Can you work these out from the model? Positions are in its coordinate system, mm. Face numbers are marked on the shaded views. Coordinates: 2 decimals unless noted, no trailing zeros. Loops run counter-clockwise (first coordinate to the right, second up) from the corner with the lowest first, then second, coordinate; pieces in that order, holes last. Notation, with made-up numbers: M -15.5,28.5 L 6.5,28.5 A23 cw 6.5,51.5 Z; hole C -21,77 d8. An arc over 180 degrees is marked long. Return JSON: item names as keys, results as strings. Group by question number.
Autodesk Inventor part; units mm, degrees
ref_plane "YZ Plane" through (0, 0, 0) normal (1, 0, 0) x (0, 1, 0)
ref_plane "XZ Plane" through (0, 0, 0) normal (0, 1, 0) x (-1, 0, 0)
ref_plane "XY Plane" through (0, 0, 0) normal (0, 0, 1) x (1, 0, 0)
sketch "skirt" plane through (0, 0, 0) normal (0, 0, 1) x (1, 0, 0)
  circle A0 centre (5.0031, 25.9038) radius 4.7625
  line L0 (24.0531, -155.0712) -> (24.0531, 181.4788)
  line L1 (-25.1594, 151.6004) -> (-25.1594, -125.1928)
  circle A1 centre (11.3531, 133.8538) radius 2.1844
  arc A2 (24.0531, 181.4788) -> (20.8781, 184.6538) centre (20.8781, 181.4788) ccw
  line L2 (20.8781, 184.6538) -> (-7.3651, 184.6538)
  line L3 (-24.646, 154.1018) -> (-13.2017, 180.8052)
  arc A3 (-7.3651, 184.6538) -> (-13.2017, 180.8052) centre (-7.3651, 178.3038) ccw
  arc A4 (-24.646, 154.1018) -> (-25.1594, 151.6004) centre (-18.8094, 151.6004) ccw
  line L4 (-24.646, -127.6942) -> (-13.2017, -154.3976)
  line L5 (-7.3651, -158.2462) -> (20.8781, -158.2462)
  arc A5 (20.8781, -158.2462) -> (24.0531, -155.0712) centre (20.8781, -155.0712) ccw
  arc A6 (-25.1594, -125.1928) -> (-24.646, -127.6942) centre (-18.8094, -125.1928) ccw
  circle A7 centre (11.3531, -120.1462) radius 2.1844
  arc A8 (-13.2017, -154.3976) -> (-7.3651, -158.2462) centre (-7.3651, -151.8962) ccw
  circle A9 centre (5.0031, 64.0038) radius 4.7625
  circle A10 centre (5.0031, 38.6038) radius 4.7625
  circle A11 centre (5.0031, 0.5038) radius 4.7625
  circle A12 centre (11.3531, -31.2462) radius 2.1844
  circle A13 centre (5.0031, -62.9962) radius 4.7625
  circle A14 centre (5.0031, -88.3962) radius 4.7625
  circle A15 centre (5.0031, 89.4038) radius 2.1844
  point P0 (-0.9322, -0.2017)
  point P1 (5.0031, 51.3038)
  point P2 (-25.1594, 152.9038)
  point P3 (-25.1594, -126.4962)
  point P4 (5.0031, -12.1962)
  point P5 (5.0031, 13.2038)
  dimension "d0" = 279.4
  dimension "d1" = 49.2125
  dimension "d2" = 3.175
  dimension "d3" = 113.199
  dimension "d4" = 113.199
  dimension "d5" = 6.35
  dimension "d7" = 9.525
  dimension "d13" = 50.8
  dimension "d14" = 38.1
  dimension "d16" = 4.3688
  dimension "d17" = 31.75
  dimension "d18" = 4.3688
sketch "Sketch1" plane through (0, 0, 0) normal (1, 0, 0) x (0, 1, 0)
  circle A0 centre (-6.35, -107.95) radius 4.7625
  line L0 (12.7, -288.925) -> (12.7, 47.625)
  line L1 (-36.5125, 17.7466) -> (-36.5125, -259.0466)
  circle A1 centre (0, 0) radius 2.1844
  arc A2 (12.7, 47.625) -> (9.525, 50.8) centre (9.525, 47.625) ccw
  line L2 (9.525, 50.8) -> (-18.7182, 50.8)
  line L3 (-35.9991, 20.248) -> (-24.5548, 46.9514)
  arc A3 (-18.7182, 50.8) -> (-24.5548, 46.9514) centre (-18.7182, 44.45) ccw
  arc A4 (-35.9991, 20.248) -> (-36.5125, 17.7466) centre (-30.1625, 17.7466) ccw
  line L4 (-35.9991, -261.548) -> (-24.5548, -288.2514)
  line L5 (-18.7182, -292.1) -> (9.525, -292.1)
  arc A5 (9.525, -292.1) -> (12.7, -288.925) centre (9.525, -288.925) ccw
  arc A6 (-36.5125, -259.0466) -> (-35.9991, -261.548) centre (-30.1625, -259.0466) ccw
  circle A7 centre (0, -254) radius 2.1844
  arc A8 (-24.5548, -288.2514) -> (-18.7182, -292.1) centre (-18.7182, -285.75) ccw
  circle A9 centre (-6.35, -69.85) radius 4.7625
  circle A10 centre (-6.35, -95.25) radius 4.7625
  circle A11 centre (-6.35, -133.35) radius 4.7625
  circle A12 centre (0, -165.1) radius 2.1844
  circle A13 centre (-6.35, -196.85) radius 4.7625
  circle A14 centre (-6.35, -222.25) radius 4.7625
  circle A15 centre (-6.35, -44.45) radius 2.1844
extrude "Extrusion1" add sketch "Sketch1" along normal blind 1.5875
properties part number "Skirt" material "Acetal Resin, White"
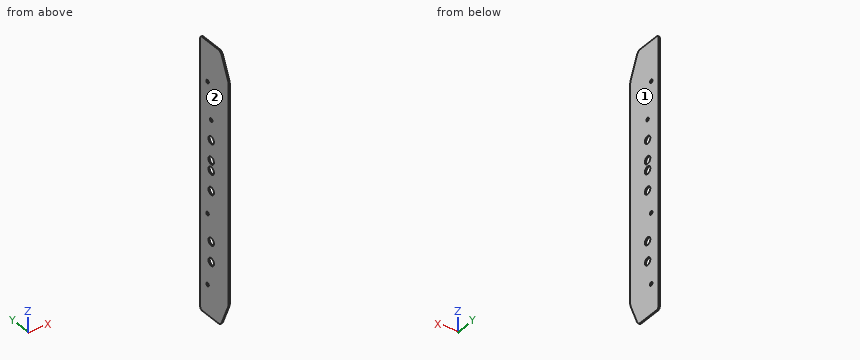
1) Suppose I cut it at A-A, the plane z = -69.85. List the corners of the cut face in (x, y) for me, then the cut area to 3 significant figures.
2) If we mould it in two halves opening along X, with no side actions, what happens to the marked faces 1 and 2? For each: +X half, -X half, draft (parallel to the pull), parting line (faces both ways), or undercut.
3) Suppose I cut it at B-B, the plane x = 0.45. Give the number of separate pieces and of enclosed holes in the cut face, then the cut area to 3 significant figures.
4) If I drill on line 1 (Y direction, x = 0.8, z = -254); line 2 (Y direction, x = 0.75, z = -99.5); line 3 (Z direction, x = 1.35, y = -32), over which ranges is the centre line in solid material (lowest first)? Write a range as from..to.
Returned:
{
 "1": {"outline": "M 0,-36.51 L 1.59,-36.51 L 1.59,-11.11 L 0,-11.11 Z; M 0,-1.59 L 1.59,-1.59 L 1.59,12.7 L 0,12.7 Z", "area": "63.0 mm²"},
 "2": {"face 1": "+X half", "face 2": "-X half"},
 "3": {"separate pieces": "1", "enclosed holes": "10", "area": "15,900 mm²"},
 "4": {"line 1": "y = -36.51..-2.18, 2.18..12.7", "line 2": "y = -36.51..-8.5, -4.2..12.7", "line 3": "z = -270.88..29.58"}
}
